```python
from build123d import *

# Parameters (mm, degrees)
SKETCH1_R           = 254.5
SKETCH1_R_2         = 234.5
BOSS_EXTRUDE1_DEPTH = 5
SKETCH2_W           = 27.805822748
SKETCH2_H           = 60
CUT_EXTRUDE1_DEPTH  = 5
SKETCH3_R           = 2.5
CUT_EXTRUDE2_DEPTH  = 5
SKETCH4_R           = 1.5
CUT_EXTRUDE3_DEPTH  = 5
SKETCH5_W           = 651.212620435
SKETCH5_H           = 357.226439325
CUT_EXTRUDE4_DEPTH  = 10
CUT_EXTRUDE9_START  = -10
SKETCH6_R           = 1.5
SKETCH6_R_2         = 2.5
CUT_EXTRUDE9_DEPTH  = 10
SKETCH7_R           = 2.5
SKETCH7_R_2         = 1.5
CUT_EXTRUDE11_DEPTH = 10


with BuildPart() as part:
    # Sketch1 → Boss-Extrude1 (new body)
    with BuildSketch(Plane(origin=(0, 0, 0), x_dir=(1, 0, 0), z_dir=(0, 1, 0))):
        with Locations(Location((0, 0, 0), (0, 0, 270))):
            Circle(SKETCH1_R)
        with Locations(Location((0, 0, 0), (0, 0, 270))):
            Circle(SKETCH1_R_2, mode=Mode.SUBTRACT)
    extrude(amount=BOSS_EXTRUDE1_DEPTH)

    # Sketch2 → Cut-Extrude1 (cut)
    with BuildSketch(Plane(origin=(0, 5, 0), x_dir=(1, 0, 0), z_dir=(0, 1, 0))):
        with Locations((-240.597088626, 30)):
            Rectangle(SKETCH2_W, SKETCH2_H)
    cut_extrude1 = extrude(amount=-CUT_EXTRUDE1_DEPTH, mode=Mode.SUBTRACT)

    # Mirror1: Cut-Extrude1 across plane
    add(cut_extrude1.mirror(Plane.XY), mode=Mode.SUBTRACT)

    # Sketch3 → Cut-Extrude2 (cut)
    with BuildSketch(Plane(origin=(0, 5, 0), x_dir=(1, 0, 0), z_dir=(0, 1, 0))):
        with Locations(Location((242.5, 0, 0), (0, 0, 270))):
            Circle(SKETCH3_R)
        with Locations(Location((196.186621136, -142.537923681, 0), (0, 0, 270))):
            Circle(SKETCH3_R)
        with Locations(Location((74.936621136, -230.631205202, 0), (0, 0, 270))):
            Circle(SKETCH3_R)
        with Locations(Location((-74.936621136, -230.631205202, 0), (0, 0, 270))):
            Circle(SKETCH3_R)
        with Locations(Location((-196.186621136, -142.537923681, 0), (0, 0, 270))):
            Circle(SKETCH3_R)
        with Locations((-242.5, 0)):
            Circle(SKETCH3_R)
        with Locations(Location((-196.186621136, 142.537923681, 0), (0, 0, 270))):
            Circle(SKETCH3_R)
        with Locations(Location((-74.936621136, 230.631205202, 0), (0, 0, 270))):
            Circle(SKETCH3_R)
        with Locations(Location((74.936621136, 230.631205202, 0), (0, 0, 270))):
            Circle(SKETCH3_R)
        with Locations(Location((196.186621136, 142.537923681, 0), (0, 0, 270))):
            Circle(SKETCH3_R)
    extrude(amount=-CUT_EXTRUDE2_DEPTH, mode=Mode.SUBTRACT)

    # Sketch4 → Cut-Extrude3 (cut)
    with BuildSketch(Plane(origin=(0, 5, 0), x_dir=(1, 0, 0), z_dir=(0, 1, 0))):
        with Locations(Location((0, -242.5, 0), (0, 0, 270))):
            Circle(SKETCH4_R)
        with Locations(Location((-142.537923681, -196.186621136, 0), (0, 0, 270))):
            Circle(SKETCH4_R)
        with Locations(Location((-230.631205202, -74.936621136, 0), (0, 0, 270))):
            Circle(SKETCH4_R)
        with Locations(Location((-230.631205202, 74.936621136, 0), (0, 0, 270))):
            Circle(SKETCH4_R)
        with Locations(Location((-142.537923681, 196.186621136, 0), (0, 0, 270))):
            Circle(SKETCH4_R)
        with Locations(Location((0, 242.5, 0), (0, 0, 270))):
            Circle(SKETCH4_R)
        with Locations(Location((142.537923681, 196.186621136, 0), (0, 0, 270))):
            Circle(SKETCH4_R)
        with Locations(Location((230.631205202, 74.936621136, 0), (0, 0, 270))):
            Circle(SKETCH4_R)
        with Locations(Location((230.631205202, -74.936621136, 0), (0, 0, 270))):
            Circle(SKETCH4_R)
        with Locations(Location((142.537923681, -196.186621136, 0), (0, 0, 270))):
            Circle(SKETCH4_R)
    extrude(amount=-CUT_EXTRUDE3_DEPTH, mode=Mode.SUBTRACT)

    # Sketch5 → Cut-Extrude4 (cut)
    with BuildSketch(Plane(origin=(0, 5, 0), x_dir=(1, 0, 0), z_dir=(0, 1, 0))):
        with Locations((-71.106310217, -178.613219663)):
            Rectangle(SKETCH5_W, SKETCH5_H)
    extrude(amount=-CUT_EXTRUDE4_DEPTH, mode=Mode.SUBTRACT)

    # Sketch6 → Cut-Extrude9 (cut)
    # profile 1 of 2: a face of its own
    with BuildSketch(Plane(origin=(0, 5, 0), x_dir=(1, 0, 0), z_dir=(0, 1, 0)).offset(CUT_EXTRUDE9_START)):
        with BuildLine():
            Line((-117.25, 203.082957187), (-127.25, 220.403465263))
            ThreePointArc((-127.25, 220.403465263), (-203.737945948, 152.51589878), (-247.326201604, 60))
            Line((-247.326201604, 60), (-226.694177252, 60))
            ThreePointArc((-226.694177252, 60), (-186.259449225, 142.469883043), (-117.25, 203.082957187))
        make_face()
        with Locations((-230.631205202, 74.936621136)):
            Circle(SKETCH6_R, mode=Mode.SUBTRACT)
        with Locations((-196.186621136, 142.537923681)):
            Circle(SKETCH6_R_2, mode=Mode.SUBTRACT)
        with Locations((-142.537923681, 196.186621136)):
            Circle(SKETCH6_R, mode=Mode.SUBTRACT)
    # profile 2 of 2: a face of its own
    with BuildSketch(Plane(origin=(0, 5, 0), x_dir=(1, 0, 0), z_dir=(0, 1, 0)).offset(CUT_EXTRUDE9_START)):
        with BuildLine():
            Line((-254.5, 0), (0, 0))
            Line((0, 0), (-117.25, 203.082957187))
            ThreePointArc((-117.25, 203.082957187), (-186.259449225, 142.469883043), (-226.694177252, 60))
            Line((-226.694177252, 60), (-247.326201604, 60))
            ThreePointArc((-247.326201604, 60), (-252.700186296, 30.213669851), (-254.5, 0))
        make_face()
    extrude(amount=CUT_EXTRUDE9_DEPTH, mode=Mode.SUBTRACT)

    # Sketch7 → Cut-Extrude11 (cut)
    # profile 1 of 2: a face of its own
    with BuildSketch(Plane(origin=(0, 5, 0), x_dir=(1, 0, 0), z_dir=(0, 1, 0))):
        with BuildLine():
            Line((99.103982378, 212.52917606), (107.556347613, 230.655331801))
            ThreePointArc((107.556347613, 230.655331801), (-11.101134084, 254.257772393), (-127.25, 220.403465263))
            Line((-127.25, 220.403465263), (-117.25, 203.082957187))
            ThreePointArc((-117.25, 203.082957187), (-10.228746337, 234.276807961), (99.103982378, 212.52917606))
        make_face()
        with Locations((-74.936621136, 230.631205202)):
            Circle(SKETCH7_R, mode=Mode.SUBTRACT)
        with Locations((0, 242.5)):
            Circle(SKETCH7_R_2, mode=Mode.SUBTRACT)
        with Locations((74.936621136, 230.631205202)):
            Circle(SKETCH7_R, mode=Mode.SUBTRACT)
    # profile 2 of 2: a face of its own
    with BuildSketch(Plane(origin=(0, 5, 0), x_dir=(1, 0, 0), z_dir=(0, 1, 0))):
        with BuildLine():
            Line((-117.25, 203.082957187), (0, 0))
            Line((0, 0), (99.103982378, 212.52917606))
            ThreePointArc((99.103982378, 212.52917606), (-10.228746337, 234.276807961), (-117.25, 203.082957187))
        make_face()
    extrude(amount=-CUT_EXTRUDE11_DEPTH, mode=Mode.SUBTRACT)


solid = part.part
```
Verification items for the finished model (mm, model axes). Round coordinates to 2 decimals unless told otherwise and drop trailing zeros. Order: outer loops, then holes, each group sorted by start corner. A loop starts at its lowest first (then second) coordinate and runs counter-clockwise, first axis right, second up.
1) Cross-section at C-C, the plane x = 154.5. Record the cut outline in (y, z).
Geometry says:
outline: (0, -202.24) - (5, -202.24) - (5, -176.41) - (0, -176.41) - close
2) Cross-section at B-B, the plane z = -136. Record the cut outline in (x, y).
Geometry says:
outline: (191.03, 0) - (215.11, 0) - (215.11, 5) - (191.03, 5) - close
3) Cross-section at A-A, the plane y = 3.6. Record the cut outline in (x, z).
Geometry says:
outline: (99.1, -212.53) - (107.56, -230.66) arc R254.5 ccw to (254.5, 0) - (245, 0) arc R2.5 cw to (240, 0) - (234.5, 0) arc R234.5 cw to start; hole circle Ø3 at (142.54, -196.19); hole circle Ø5 at (196.19, -142.54); hole circle Ø3 at (230.63, -74.94)
4) Depth check by flat-ended pin: pin 1 (2 mm diameter, centred on x = 168, y = 4.5, fed in from +Z); pin 2 (1.5 mm diameter, centred on y = 2.5, z = -51, fed in from -X); pin 3 (1.5 mm diameter, centred on x = 204.5, y = 0.5, fed in from +Z). Enter the tip coordinate at first touch or a pass-through.
Geometry says:
pin 1: stops at z = -162.57
pin 2: stops at x = 228.72
pin 3: stops at z = -113.41
5) Draft check along X on faces 1 (the cylindrical face through (194.665, 2.535, -144.522)), 2 (the flat face through (103.271, 2.535, -221.465)), 3 (the flat face through (200, 5, -124)). Enter one of: +X half, -X half, draft (parallel to the pull), parting line (faces both ways), or undercut.
Geometry says:
face 1: undercut
face 2: -X half
face 3: draft
6) Material ranges on line 1 (X direction, y = 4.2, z = -197); line 2 (Z direction, x = 162.5, y = 1.9); line 3 (Z direction, x = 218, y = 1.45), recorded low to high.
Geometry says:
line 1: x = 127.21 to 141.28, 143.8 to 161.12
line 2: z = -195.87 to -169.07
line 3: z = -131.32 to -86.41
